Check sheet for the modelled part. Datum: model origin and axes. Units: mm. A direction names the side the tool comes from. Coordinates: 2 decimals unless noted, no trailing zeros. Write each loop counter-clockwise with the first axis right and the second up, starting at its lowest first coordinate (ties: lowest second). Pieces come first, ordered by that corner, then holes. Notation, with made-up numbers: (25.25, -2) - (34.25, -2) arc R17 ccw to (34.25, 31) - close; hole circle Ø1 at (17, -37.75). An arc over 180 degrees is marked (long way). Use one line per item in the form item = value. Start each with the question number.
1. Go/stop test with flat-tipped pins: pin 1 Ø5 at (x, z) = (-11, -9) entering from +Y; pin 2 Ø3 at (y, z) = (-24, -4) entering from -X; pin 3 Ø3.5 at (x, y) = (-5, -34.75) entering from +Z; pin 4 Ø3 at (x, z) = (16, -3) entering from -Y. Record where each tip stops, or that it passes through.
2. Scan lines: line 1 along Y through (x, z) = (-5.5, -6); line 2 along Y through (x, z) = (3.5, -16); line 3 along X through (y, z) = (-2, -14.5). Record each from-to range of solid material in increasing order.
3. Cross-section at C-C on y = 26.25. Record the boundary of the cut face in (x, z).
4. Cross-section at B-B on y = 0. Record the boundary of the cut face in (x, z), then the cut area to 3 significant figures.
5. Draft check along Y on faces 6 (the face through (-2.414, 16.271, -12.112)), 7 (the face through (-8, 26, -10)), 8 (the face through (5, -37.75, -12)). Enter one of: +Y half, -Y half, draft (parallel to the pull), parting line (faces both ways), or undercut.
6. Cross-section at D-D on x = -12. Record the boundary of the cut face in (y, z), then the cut area to 3 significant figures.
7. Cross-section at A-A on x = 5. Record the boundary of the cut face in (y, z), then the cut area to 3 significant figures.
8. Tool access check on faces 1 (the face through (14.54, 5.82, -6.58)), 2 (the face through (-16.077, 5.43, -13.424)), 3 (the face through (-14, 0, -7)), 4 (the face through (0, -30.1, -10)), 5 (the face through (-7.586, 13.229, -12.112)). Record the directions out of +Z, -Z, +X, -X, +Y, -Y that give a thin tool (end or side, any length) a straight path to the whole face; none if there is none.
```python
from build123d import *

# Parameters (mm, degrees)
SKETCH1_W                                           = 40
SKETCH1_H                                           = 70.5
BOSS_EXTRUDE1_DEPTH                                 = 20
SKETCH2_W                                           = 20.2
SKETCH2_H                                           = 40.2
CUT_EXTRUDE1_DEPTH                                  = 30
CBORE_FOR_M3_HEX_SOCKET_HEAD_CAP_SCREW1_D           = 3.2
CBORE_FOR_M3_HEX_SOCKET_HEAD_CAP_SCREW1_DEPTH       = 7.9
CBORE_FOR_M3_HEX_SOCKET_HEAD_CAP_SCREW1_CBORE_D     = 6.5
CBORE_FOR_M3_HEX_SOCKET_HEAD_CAP_SCREW1_CBORE_DEPTH = 4
CUT_EXTRUDE2_DEPTH                                  = 9
SKETCH8_R                                           = 4.5
CUT_EXTRUDE3_DEPTH                                  = 58.593163657
CUT_EXTRUDE4_DEPTH                                  = 50.239846669
CUT_EXTRUDE4_DEPTH_BACK                             = 50.239846669
SKETCH12_R                                          = 2
CUT_EXTRUDE5_DEPTH                                  = 50.239846669
CUT_EXTRUDE6_DEPTH                                  = 16
SKETCH15_W                                          = 10
SKETCH15_H                                          = 10
CUT_EXTRUDE7_DEPTH                                  = 50.239846669
SKETCH16_R                                          = 1.75
CUT_EXTRUDE8_DEPTH                                  = 54.296927679
CUT_EXTRUDE9_REACH                                  = 61.503
SKETCH17_R                                          = 3


with BuildPart() as part:
    # Sketch1 → Boss-Extrude1 (new body)
    with BuildSketch(Plane.XY):
        with Locations((2, -4)):
            Rectangle(SKETCH1_W, SKETCH1_H)
    extrude(amount=-BOSS_EXTRUDE1_DEPTH)

    # Sketch2 → Cut-Extrude1 (cut)
    with BuildSketch(Plane.XY):
        with Locations((0, -10)):
            Rectangle(SKETCH2_W, SKETCH2_H)
    extrude(amount=-CUT_EXTRUDE1_DEPTH, mode=Mode.SUBTRACT)

    # CBORE for M3 Hex Socket Head Cap Screw1
    with Locations(Plane(origin=(-10.1, 0, 0), x_dir=(0, 0, -1), z_dir=(1, 0, 0))):
        with Locations((5.050252532, 4.949747468), (14.949747468, 4.949747468), (14.949747468, -4.949747468), (5.050252532, -4.949747468)):
            CounterBoreHole(CBORE_FOR_M3_HEX_SOCKET_HEAD_CAP_SCREW1_D / 2, CBORE_FOR_M3_HEX_SOCKET_HEAD_CAP_SCREW1_CBORE_D / 2, CBORE_FOR_M3_HEX_SOCKET_HEAD_CAP_SCREW1_CBORE_DEPTH, depth=CBORE_FOR_M3_HEX_SOCKET_HEAD_CAP_SCREW1_DEPTH)

    # Sketch7 → Cut-Extrude2 (cut)
    with BuildSketch(Plane.ZY.offset(-10.1)):
        Polygon((-10, 7.794228634), (-16.75, 3.897114317), (-16.75, -3.897114317), (-10, -7.794228634), (-3.25, -3.897114317), (-3.25, 3.897114317), align=None)
    extrude(amount=-CUT_EXTRUDE2_DEPTH, mode=Mode.SUBTRACT)

    # Sketch8 → Cut-Extrude3 (cut, through all)
    with BuildSketch(Plane.ZY.offset(-19.1)):
        with Locations(Location((-10, 0, 0), (0, 0, 270))):
            Circle(SKETCH8_R)
    extrude(amount=-CUT_EXTRUDE3_DEPTH, mode=Mode.SUBTRACT)

    # Sketch9 → Cut-Extrude4 (cut, two sides: drawn at the far end of the back side and taken through both)
    with BuildSketch(Plane.XY.offset(-CUT_EXTRUDE4_DEPTH_BACK)):
        Polygon((-18, -10), (-10, -39.25), (-18, -39.25), align=None)
        Polygon((10, -39.25), (22, -10), (22, -39.25), align=None)
    extrude(amount=CUT_EXTRUDE4_DEPTH + CUT_EXTRUDE4_DEPTH_BACK, mode=Mode.SUBTRACT)

    # Sketch12 → Cut-Extrude5 (cut, through all)
    with BuildSketch(Plane.XY):
        with Locations((-5, -34.75)):
            Circle(SKETCH12_R)
        with Locations((5, -34.75)):
            Circle(SKETCH12_R)
        with Locations((5, 14.75)):
            Circle(SKETCH12_R)
        with Locations((-5, 14.75)):
            Circle(SKETCH12_R)
    extrude(amount=-CUT_EXTRUDE5_DEPTH, mode=Mode.SUBTRACT)

    # Sketch13 → Cut-Extrude6 (cut)
    with BuildSketch(Plane(origin=(0, 0, -20), x_dir=(-1, 0, 0), z_dir=(0, 0, -1))):
        Polygon((-1.535898385, 14.75), (-3.267949192, 17.75), (-6.732050808, 17.75), (-8.464101615, 14.75), (-6.732050808, 11.75), (-3.267949192, 11.75), align=None)
        Polygon((3.267949192, 17.75), (1.535898385, 14.75), (3.267949192, 11.75), (6.732050808, 11.75), (8.464101615, 14.75), (6.732050808, 17.75), align=None)
        Polygon((-6.732050808, -31.75), (-8.464101615, -34.75), (-6.732050808, -37.75), (-3.267949192, -37.75), (-1.535898385, -34.75), (-3.267949192, -31.75), align=None)
        Polygon((3.267949192, -31.75), (1.535898385, -34.75), (3.267949192, -37.75), (6.732050808, -37.75), (8.464101615, -34.75), (6.732050808, -31.75), align=None)
    extrude(amount=-CUT_EXTRUDE6_DEPTH, mode=Mode.SUBTRACT)

    # Sketch15 → Cut-Extrude7 (cut, through all)
    with BuildSketch(Plane.XY):
        with Locations((-13, 26.25)):
            Rectangle(SKETCH15_W, SKETCH15_H)
        with Locations((17, 26.25)):
            Rectangle(SKETCH15_W, SKETCH15_H)
    extrude(amount=-CUT_EXTRUDE7_DEPTH, mode=Mode.SUBTRACT)

    # Sketch16 → Cut-Extrude8 (cut, through all)
    with BuildSketch(Plane.ZY.offset(8)):
        with Locations((-16, 26.25)):
            Circle(SKETCH16_R)
        with Locations((-4, 26.25)):
            Circle(SKETCH16_R)
    extrude(amount=-CUT_EXTRUDE8_DEPTH, mode=Mode.SUBTRACT)

    # Sketch17 → Cut-Extrude9 (cut, up to next)
    with BuildSketch(Plane.ZY.offset(18), mode=Mode.PRIVATE) as cut_extrude9_sk1:
        with Locations(Location((-10, 0, 0), (0, 0, 270))):
            Circle(SKETCH17_R)
    cut_extrude9_tool1 = extrude(cut_extrude9_sk1.sketch, amount=-CUT_EXTRUDE9_REACH, mode=Mode.PRIVATE) & part.part
    add(cut_extrude9_tool1.solids().sort_by_distance((-18, 0, -10))[0], mode=Mode.SUBTRACT)


solid = part.part
```
Final values:
q1.pin_1 = 21.25
q1.pin_2 = -14.58
q1.pin_3 = through
q1.pin_4 = -28.28
q2.line_1 = -39.25 to -37.75, -31.75 to -30.1, 10.1 to 11.75, 17.75 to 31.25
q2.line_2 = -39.25 to -37.75, -31.75 to -30.1, 10.1 to 11.75, 17.75 to 24.5, 28 to 31.25
q2.line_3 = -18 to -14.1, 19.1 to 22
q3.outline = (-8, -20) - (12, -20) - (12, -17.75) - (-8, -17.75) - close; (-8, -14.25) - (12, -14.25) - (12, -5.75) - (-8, -5.75) - close; (-8, -2.25) - (12, -2.25) - (12, 0) - (-8, 0) - close
q4.outline = (-18, -20) - (-10.1, -20) - (-10.1, -13) - (-18, -13) - close; (-18, -7) - (-10.1, -7) - (-10.1, 0) - (-18, 0) - close; (10.1, -20) - (22, -20) - (22, -14.5) - (19.1, -14.5) - (19.1, -16.75) - (10.1, -16.75) - close; (10.1, -3.25) - (19.1, -3.25) - (19.1, -5.5) - (22, -5.5) - (22, 0) - (10.1, 0) - close
q4.area = 201 mm²
q5.face_6 = undercut
q5.face_7 = draft
q5.face_8 = undercut
q6.outline = (-31.94, -20) - (21.25, -20) - (21.25, 0) - (-31.94, 0) - close; hole circle Ø6.5 at (-4.95, -14.95); hole circle Ø6.5 at (-4.95, -5.05); hole circle Ø6 at (0, -10); hole circle Ø6.5 at (4.95, -14.95); hole circle Ø6.5 at (4.95, -5.05)
q6.area = 903 mm²
q7.outline = (-39.25, -20) - (-37.75, -20) - (-37.75, -4) - (-36.75, -4) - (-36.75, 0) - (-39.25, 0) - close; (-32.75, -4) - (-31.75, -4) - (-31.75, -20) - (-30.1, -20) - (-30.1, 0) - (-32.75, 0) - close; (10.1, -20) - (11.75, -20) - (11.75, -4) - (12.75, -4) - (12.75, 0) - (10.1, 0) - close; (16.75, -4) - (17.75, -4) - (17.75, -20) - (31.25, -20) - (31.25, 0) - (16.75, 0) - close; hole circle Ø3.5 at (26.25, -16); hole circle Ø3.5 at (26.25, -4)
q7.area = 363 mm²
q8.face_1 = none
q8.face_2 = -X
q8.face_3 = +X, -X
q8.face_4 = +Z, -Z
q8.face_5 = -Z
